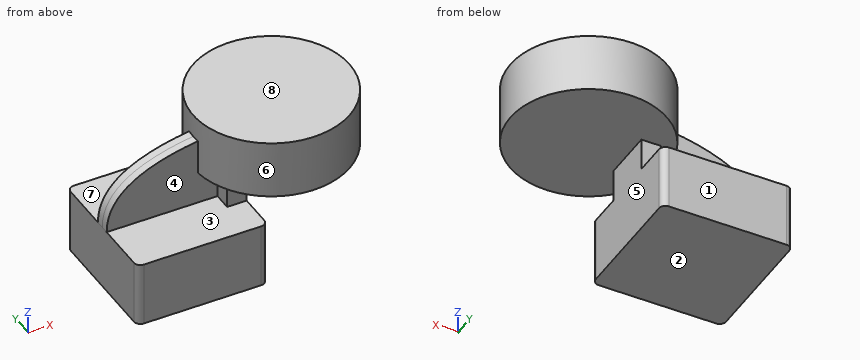
```python
from build123d import *

# Parameters (mm, degrees)
F1_DEPTH = 63.5
F0_W     = 19.994952
F0_H     = 19.05
F2_DEPTH = 25.4
F3_DEPTH = 7.9375
F5_R     = 6.35


with BuildPart() as f1:
    # F0 (on Front) → F1 (new body, symmetric)
    with BuildSketch(Plane.XZ):
        Polygon((-127, 0), (0, 0), (0, 63.5), (-19.05, 63.5), (-127, 63.5), align=None)
    extrude(amount=F1_DEPTH, both=True)

    # F0 (on Front) → F2 (join, symmetric)
    with BuildSketch(Plane.XZ):
        with BuildLine():
            Line((-19.05, 63.5), (0, 63.5))
            Line((0, 63.5), (0, 98.425))
            ThreePointArc((0, 98.425), (4.64968, 109.65032), (15.875, 114.3))
            Line((15.875, 114.3), (37.741059, 114.3))
            Line((37.741059, 114.3), (37.741059, 133.35))
            Line((37.741059, 133.35), (15.875, 133.35))
            add(Edge.make_bspline(
                [(15.151937, 133.342514), (15.39375, 133.34518), (15.634775, 133.347673), (15.875, 133.35)],
                knots=[158.307474, 158.307474, 158.307474, 158.307474, 159.035493, 159.035493, 159.035493, 159.035493], degree=3))
            ThreePointArc((15.151937, 133.342514), (-9.075036, 122.863726), (-19.05, 98.425))
            Line((-19.05, 98.425), (-19.05, 63.5))
        make_face()
        with Locations((47.738535, 123.825)):
            Rectangle(F0_W, F0_H)
    extrude(amount=F2_DEPTH, both=True)

    # F0 (on Front) → F3 (join, symmetric)
    with BuildSketch(Plane.XZ):
        with BuildLine():
            add(Edge.make_bspline(
                [(-127, 63.5), (-127.275289, 124.073074), (-37.430264, 132.762938), (15.151937, 133.342514)],
                knots=[0, 0, 0, 0, 158.307474, 158.307474, 158.307474, 158.307474], degree=3))
            Line((-127, 63.5), (-19.05, 63.5))
            Line((-19.05, 63.5), (-19.05, 98.425))
            ThreePointArc((-19.05, 98.425), (-9.075036, 122.863726), (15.151937, 133.342514))
        make_face()
    extrude(amount=F3_DEPTH, both=True)

    # F0 (on Front) → F4 (revolve)
    with BuildSketch(Plane.XZ):
        Polygon((57.736011, 114.3), (37.741059, 114.3), (37.741059, 95.25), (113.941059, 95.25), (113.941059, 152.4), (37.741059, 152.4), (37.741059, 133.35), (57.736011, 133.35), align=None)
    revolve(axis=Axis((37.741059, 0, 123.825), (0, 0, 1)))

    # F5
    f5_edges = [f1.edges().sort_by_distance(p)[0] for p in [
        (-127, -63.5, 31.75),
        (0, -63.5, 31.75),
        (-127, 63.5, 31.75),
        (0, 63.5, 31.75),
    ]]
    fillet(f5_edges, radius=F5_R)


solid = f1.part
```
Can you work these out from the model? Positions are in its coordinate system, mm. Face numbers are marked on the shaded views. A direction names the side the tool comes from. Coordinates: 2 decimals unless noted, no trailing zeros. Loops run counter-clockwise (first coordinate to the right, second up) from the corner with the lowest first, then second, coordinate; pieces in that order, holes last. Notation, with made-up numbers: (22, 76.5) - (79, 76.5) arc R21 cw to (79, 115.5) - close; hole circle Ø9 at (56.25, 13). An arc over 180 degrees is marked (long way). Answer as CSV lines item,"result". Start each with the question number.
1) I need wall thicknesses on line 1 (Z direction, x = -22.5, y = 45); line 2 (Z direction, x = 36, y = 29.5); line 3 (X direction, y = 14, z = 38.5). Which ranges of each line are inside material? Lowest first, please. Write a range as from..to.
2) Thinking about a two-plate mould opening in Z: for the marked faces 1, 2 and 3, which applies, pulls with the +Z half, pulls with the -Z half, needs draft (parallel to the pull), parting line crosses it, or undercut?
3) For pin 1 (21 mm diameter, centred on x = -10.5, z = 72.5, fed in from -Y); pin 2 (1.5 mm diameter, centred on y = 3, z = 79, fed in from +X); pin 3 (2 mm diameter, centred on x = -101.5, z = 29.5, fed in from +Y), each with a flat end and sliding along its axis, tell me the tip position at first contact or that it passes through.
4) Suppose I cut it at B-B (z = 50). Please give me the cut outline in (x, y).
5) Suppose I cut it at C-C (y = -50.5). Please give me the cut outline in (x, z).
6) Suppose I cut it at D-D (x = 34). Please give me the cut outline in (y, z), plus the area to 3 significant figures.
7) Suppose I cut it at A-A (y = 43.5). Please give me the cut outline in (x, z).
8) Which directions (+Z, -Z, +X, -X, +Y, -Y) give clear straight access to the entire face, cutting with the end or side of a thin tool? Please do the marked faces 4, 5, 6, 7 and 8.
Check result:
1,line 1,"z = 0..63.5, 95.25..152.4"
1,line 2,"z = 95.25..152.4"
1,line 3,"x = -127..0"
2,face 1,"needs draft"
2,face 2,"pulls with the -Z half"
2,face 3,"undercut"
3,pin 1,"stops at y = -63.5"
3,pin 2,"stops at x = 0"
3,pin 3,"stops at y = 63.5"
4,outline,"(-127, -57.15) arc R6.35 ccw to (-120.65, -63.5) - (-6.35, -63.5) arc R6.35 ccw to (0, -57.15) - (0, 57.15) arc R6.35 ccw to (-6.35, 63.5) - (-120.65, 63.5) arc R6.35 ccw to (-127, 57.15) - close"
5,outline,"(-127, 0) - (0, 0) - (0, 63.5) - (-127, 63.5) - close; (-19.32, 95.25) - (94.8, 95.25) - (94.8, 152.4) - (-19.32, 152.4) - close"
6,outline,"(-76.11, 95.25) - (76.11, 95.25) - (76.11, 152.4) - (-76.11, 152.4) - close"
6,area,"8,700 mm²"
7,outline,"(-127, 0) - (0, 0) - (0, 63.5) - (-127, 63.5) - close; (-24.82, 95.25) - (100.3, 95.25) - (100.3, 152.4) - (-24.82, 152.4) - close"
8,face 4,"-X, -Y"
8,face 5,"-Z, +X, +Y, -Y"
8,face 6,"+Z"
8,face 7,"-X, +Y"
8,face 8,"+Z, +X, -X, +Y, -Y"
